```python
from build123d import *

# Parameters (mm, degrees)
BOSS_EXTRUDE1_DEPTH     = 3.175
SKETCH2_W               = 3.175
SKETCH2_H               = 38.1
BOSS_EXTRUDE2_DEPTH     = 41.275
SKETCH3_W               = 44.45
SKETCH3_H               = 22.225
BOSS_EXTRUDE3_DEPTH     = 76.2
SCALE1_SCALE            = 1.333333333
CUT_EXTRUDE2_DEPTH      = 132.738543571
CUT_EXTRUDE2_DEPTH_BACK = 132.738543571
CUT_EXTRUDE3_DEPTH      = 127.255434571
CUT_EXTRUDE3_DEPTH_BACK = 127.255434571
SKETCH6_R               = 3.175
CUT_EXTRUDE4_DEPTH      = 132.738543571
CUT_EXTRUDE4_DEPTH_BACK = 132.738543571
SKETCH7_R               = 3.175
CUT_EXTRUDE5_DEPTH      = 118.143916866
CUT_EXTRUDE5_DEPTH_BACK = 118.143916866
SKETCH8_R               = 3.175


with BuildPart() as part:
    # Sketch1 → Boss-Extrude1 (new body)
    with BuildSketch(Plane.XY):
        Polygon((0, 0), (38.1, 0), (76.2, 38.1), (0, 38.1), align=None)
    boss_extrude1 = extrude(amount=BOSS_EXTRUDE1_DEPTH)

    # Sketch2 → Boss-Extrude2 (add)
    with BuildSketch(Plane.XY.offset(3.175)):
        with Locations((1.5875, 19.05)):
            Rectangle(SKETCH2_W, SKETCH2_H)
    extrude(amount=BOSS_EXTRUDE2_DEPTH)

    # Mirror1: Boss-Extrude1 across plane
    add(boss_extrude1.mirror(Plane.XY.offset(22.225)))

    # Sketch3 → Boss-Extrude3 (add)
    with BuildSketch(Plane.ZY):
        with Locations((22.225, 49.2125)):
            Rectangle(SKETCH3_W, SKETCH3_H)
    extrude(amount=-BOSS_EXTRUDE3_DEPTH)


with BuildPart() as part_1:
    # Scale1: scaled about (35.055122951, 43.591188525, 22.225)
    add(part.part.scale(SCALE1_SCALE).moved(Location((-11.685040984, -14.530396175, -7.408333333))))

    # Sketch5 → Cut-Extrude2 (cut, two sides: drawn at the far end of the back side and taken through both)
    with BuildSketch(Plane.ZY.offset(11.685040984).offset(-CUT_EXTRUDE2_DEPTH_BACK)):
        Polygon((28.575, 55.461540547), (22.225, 59.127714756), (15.875, 55.461540547), (15.875, 48.129192128), (22.225, 44.463017919), (28.575, 48.129192128), align=None)
    extrude(amount=CUT_EXTRUDE2_DEPTH + CUT_EXTRUDE2_DEPTH_BACK, mode=Mode.SUBTRACT)

    # Sketch6 → Cut-Extrude3 (cut, two sides: drawn at the far end of the back side and taken through both)
    with BuildSketch(Plane(origin=(0, 0, -7.408333333), x_dir=(-1, 0, 0), z_dir=(0, 0, -1)).offset(-CUT_EXTRUDE3_DEPTH_BACK)):
        with Locations((-1.014959016, 23.569603825)):
            Circle(SKETCH6_R)
        with Locations((-26.414959016, -1.830396175)):
            Circle(SKETCH6_R)
    extrude(amount=CUT_EXTRUDE3_DEPTH + CUT_EXTRUDE3_DEPTH_BACK, mode=Mode.SUBTRACT)

    # Sketch7 → Cut-Extrude4 (cut, two sides: drawn at the far end of the back side and taken through both)
    with BuildSketch(Plane.ZY.offset(11.685040984).offset(-CUT_EXTRUDE4_DEPTH_BACK)):
        with Locations(Location((7.408333333, 24.386762915, 0), (0, 0, 270))):
            Circle(SKETCH7_R)
        with Locations(Location((37.041666667, -1.830396175, 0), (0, 0, 270))):
            Circle(SKETCH7_R)
    extrude(amount=CUT_EXTRUDE4_DEPTH + CUT_EXTRUDE4_DEPTH_BACK, mode=Mode.SUBTRACT)

    # Sketch8 → Cut-Extrude5 (cut, two sides: drawn at the far end of the back side and taken through both)
    with BuildSketch(Plane(origin=(0, 0, 28.575), x_dir=(-1, 0, 0), z_dir=(0, 0, -1)).offset(-CUT_EXTRUDE5_DEPTH_BACK)):
        with Locations(Location((-84.962592617, 51.795366338, 0), (0, 0, 90))):
            Circle(SKETCH8_R)
        with Locations(Location((-74.802592617, 51.795366338, 0), (0, 0, 90))):
            Circle(SKETCH8_R)
        with Locations(Location((-64.642592617, 51.795366338, 0), (0, 0, 90))):
            Circle(SKETCH8_R)
        with Locations(Location((-54.482592617, 51.795366338, 0), (0, 0, 90))):
            Circle(SKETCH8_R)
        with Locations(Location((-44.322592617, 51.795366338, 0), (0, 0, 90))):
            Circle(SKETCH8_R)
        with Locations(Location((-34.162592617, 51.795366338, 0), (0, 0, 90))):
            Circle(SKETCH8_R)
        with Locations(Location((-24.002592617, 51.795366338, 0), (0, 0, 90))):
            Circle(SKETCH8_R)
        with Locations(Location((-13.842592617, 51.795366338, 0), (0, 0, 90))):
            Circle(SKETCH8_R)
        with Locations(Location((-3.682592617, 51.795366338, 0), (0, 0, 90))):
            Circle(SKETCH8_R)
        with Locations(Location((6.477407383, 51.795366338, 0), (0, 0, 90))):
            Circle(SKETCH8_R)
    extrude(amount=CUT_EXTRUDE5_DEPTH + CUT_EXTRUDE5_DEPTH_BACK, mode=Mode.SUBTRACT)


solid = part_1.part
```
The listing builds one solid part. Answer for the finished solid, in the listing's coordinates (mm). A direction names the side the tool comes from. Coordinates: 2 decimals unless noted, no trailing zeros. Loops run counter-clockwise (first coordinate to the right, second up) from the corner with the lowest first, then second, coordinate; pieces in that order, holes last. Notation, with made-up numbers: (52, 87.5) -> (111, 87.5) arc R32 cw to (111, 114.5) -> close; hole circle Ø1 at (27.5, 74). An arc over 180 degrees is marked (long way). Use one line per item in the form item = value. Start each with the question number.
Item 1: Consider L1, parallel to Z at x = 47, y = 19 (3 decimals); L2, parallel to Z at x = 11, y = 49.5 (3 decimals); L3, parallel to X at y = 30, z = 41.5. Determine where each line is inside the solid, lowest interval first. Write a range as [from, to].
Item 2: Flat-ended cylindrical pins translate along their axes: pin 1 Ø7.5 at (y, z) = (24.39, 7.41) entering from +X; pin 2 Ø4 at (x, y) = (34.16, 51.8) entering from +Z; pin 3 Ø10 at (x, z) = (29, 34.5) entering from -Y. Find the tip coordinate at first contact, or state that the pin passes through.
Item 3: A tool of negligible diameter and unlimited length cuts with its end or side. For faces 1 (the face through (89.915, 51, 15)), 2 (the face through (39.83, 46.32, 19.01)), from which of +Z, -Z, +X, -X, +Y, -Y can it reach the whole face along a straight path? Write none if from no direction.
Item 4: The part is cut by section B-B on z = 32.5. Count the separate pieces of the cut face and the enclosed holes in it, then the cut area to 3 significant figures.
Item 5: The part is cut by section D-D on z = 18.5. Determine the outline of the cut face in (x, y), then the cut area to 3 significant figures.
Item 6: The part is cut by section A-A on x = 43. Determine the outline of the cut face in (y, z) (3 decimals), then the cut area to 3 significant figures.
Item 7: The mould has two halves that part along Z. Classify faces 3 (the face through (-9.539, -1.142, 33.942)), 4 (the face through (38, 65.903, 22)), 5 (the face through (27, 25, -7.408)): released by +Z, released by -Z, zero draft, split by the parting line, or undercut.
Answer key:
q1.L1 = [-7.408, -3.175], [47.625, 51.858]
q1.L2 = [-7.408, 15.875], [28.575, 51.858]
q1.L3 = [-11.69, -7.45]
q2.pin_1 = -7.45
q2.pin_2 = through
q2.pin_3 = 36.27
q3.face_1 = +Z, -Z, +X, +Y, -Y
q3.face_2 = +X, -X
q4.separate_pieces = 1
q4.enclosed_holes = 10
q4.area = 2,910 mm2
q5.outline = (-11.69, -14.53) -> (-7.45, -14.53) -> (-7.45, 36.27) -> (89.91, 36.27) -> (89.91, 46.61) -> (-11.69, 46.61) -> close; (-11.69, 56.98) -> (89.91, 56.98) -> (89.91, 65.9) -> (-11.69, 65.9) -> close
q5.area = 2,170 mm2
q6.outline = (-10.645, -7.408) -> (48.909, -7.408) -> (48.909, 15.875) -> (48.129, 15.875) -> (44.463, 22.225) -> (48.129, 28.575) -> (48.909, 28.575) -> (48.909, 51.858) -> (-10.645, 51.858) -> (-10.645, 47.625) -> (36.27, 47.625) -> (36.27, -3.175) -> (-10.645, -3.175) -> close; (54.682, -7.408) -> (65.903, -7.408) -> (65.903, 51.858) -> (54.682, 51.858) -> (54.682, 28.575) -> (55.462, 28.575) -> (59.128, 22.225) -> (55.462, 15.875) -> (54.682, 15.875) -> close
q6.area = 1,740 mm2
q7.face_3 = undercut
q7.face_4 = zero draft
q7.face_5 = released by -Z
